Read the model definition and answer for the solid it produces. Units are mm, in the model's axes. A direction names the side the tool comes from. Round coordinates to 2 decimals unless told otherwise and drop trailing zeros. Write each loop counter-clockwise with the first axis right and the second up, starting at its lowest first coordinate (ties: lowest second). Pieces come first, ordered by that corner, then holes.
from build123d import *

# Parameters (mm, degrees)
CROQUIS1_W              = 290
CROQUIS1_H              = 898
CROQUIS1_R              = 6
CROQUIS1_R_2            = 7
CROQUIS1_W_2            = 137.6
CROQUIS1_H_2            = 745.6
SALIENTE_EXTRUIR1_DEPTH = 50.8
REDONDEO1_R             = 5
REDONDEO2_R             = 5


with BuildPart() as part:
    # Croquis1 → Saliente-Extruir1 (new body)
    with BuildSketch(Plane(origin=(0, 0, 0), x_dir=(1, 0, 0), z_dir=(0, 1, 0))):
        with Locations((-145, 449)):
            Rectangle(CROQUIS1_W, CROQUIS1_H)
        with Locations(Location((-273.75, 375.5, 0), (0, 0, 270))):
            Circle(CROQUIS1_R, mode=Mode.SUBTRACT)
        with Locations(Location((-273.75, 522.5, 0), (0, 0, 270))):
            Circle(CROQUIS1_R, mode=Mode.SUBTRACT)
        with Locations(Location((-30.75, 377, 0), (0, 0, 270))):
            Circle(CROQUIS1_R_2, mode=Mode.SUBTRACT)
        with Locations(Location((-30.75, 521, 0), (0, 0, 270))):
            Circle(CROQUIS1_R_2, mode=Mode.SUBTRACT)
        with Locations(Location((-30.75, 167, 0), (0, 0, 270))):
            Circle(CROQUIS1_R_2, mode=Mode.SUBTRACT)
        with Locations(Location((-273.75, 732.5, 0), (0, 0, 90))):
            Circle(CROQUIS1_R, mode=Mode.SUBTRACT)
        with Locations(Location((-273.75, 312.5, 0), (0, 0, 270))):
            Circle(CROQUIS1_R, mode=Mode.SUBTRACT)
        with Locations(Location((-30.75, 311, 0), (0, 0, 270))):
            Circle(CROQUIS1_R_2, mode=Mode.SUBTRACT)
        with Locations(Location((-273.75, 165.5, 0), (0, 0, 270))):
            Circle(CROQUIS1_R, mode=Mode.SUBTRACT)
        with Locations(Location((-30.75, 587, 0), (0, 0, 90))):
            Circle(CROQUIS1_R_2, mode=Mode.SUBTRACT)
        with Locations(Location((-273.75, 585.5, 0), (0, 0, 90))):
            Circle(CROQUIS1_R, mode=Mode.SUBTRACT)
        with Locations(Location((-30.75, 731, 0), (0, 0, 90))):
            Circle(CROQUIS1_R_2, mode=Mode.SUBTRACT)
        with Locations((-145, 449)):
            Rectangle(CROQUIS1_W_2, CROQUIS1_H_2, mode=Mode.SUBTRACT)
    extrude(amount=SALIENTE_EXTRUIR1_DEPTH)

    # Redondeo1
    redondeo1_edges = [part.edges().sort_by_distance(p)[0] for p in [
        (-290, 50.8, -449),
        (-145, 50.8, 0),
        (-76.2, 50.8, -449),
        (-145, 50.8, -821.8),
        (-213.8, 50.8, -449),
        (-145, 50.8, -76.2),
        (0, 50.8, -449),
        (-145, 50.8, -898),
    ]]
    fillet(redondeo1_edges, radius=REDONDEO1_R)

    # Redondeo2
    redondeo2_edges = [part.edges().sort_by_distance(p)[0] for p in [
        (-76.2, 0, -449),
        (-145, 0, -821.8),
        (-213.8, 0, -449),
        (-145, 0, -76.2),
        (-145, 0, 0),
        (-290, 0, -449),
        (-145, 0, -898),
        (0, 0, -449),
    ]]
    fillet(redondeo2_edges, radius=REDONDEO2_R)


solid = part.part
Q1. Section A-A (z = -266) is taken. Determine the outline of the cut face in (x, y), then the cut area to 3 significant figures.
Verdict:
outline: (-290, 5) arc R5 ccw to (-285, 0) - (-218.8, 0) arc R5 ccw to (-213.8, 5) - (-213.8, 45.8) arc R5 ccw to (-218.8, 50.8) - (-285, 50.8) arc R5 ccw to (-290, 45.8) - close; (-76.2, 5) arc R5 ccw to (-71.2, 0) - (-5, 0) arc R5 ccw to (0, 5) - (0, 45.8) arc R5 ccw to (-5, 50.8) - (-71.2, 50.8) arc R5 ccw to (-76.2, 45.8) - close
area: 7,700 mm2
Q2. Determine the mould class of faces 3 (the flat face through (-240, 0, -455)), 4 (the flat face through (-213.8, 25, -444)), 5 (the flat face through (-290, 25, -443)) for opening direction X: pulls with the +X half, pulls with the -X half, needs draft (parallel to the pull), parting line crosses it, or undercut.
Verdict:
face 3: needs draft
face 4: undercut
face 5: pulls with the -X half
Q3. Straight lines are drawn through the part: probe 1 along X at (y, z) = (28, -312.5); probe 2 along X at (y, z) = (14, -522); probe 3 along X at (y, z) = (26.5, -85). For each, find the intervals that lie inside material, in ascending order.
Verdict:
probe 1: x = -290 to -279.75, -267.75 to -213.8, -76.2 to -37.59, -23.91 to 0
probe 2: x = -290 to -279.73, -267.77 to -213.8, -76.2 to -37.68, -23.82 to 0
probe 3: x = -290 to -213.8, -76.2 to 0
Q4. Section B-B (y = 25.5) is taken. State how many separate pieces and enclosed holes the cut face has, then the cut area to 3 significant figures.
Verdict:
separate pieces: 1
enclosed holes: 13
area: 156,000 mm2
Q5. Which of the six approach directions +Z, -Z, +X, -X, +Y, -Y give full straight-line access (tool end or side, diameter ignored) to faces 1 (the flat face through (-146, 25, -821.8)), 2 (the flat face through (-147, 25, -898))?
Verdict:
face 1: +Y, -Y
face 2: -Z, +X, -X, +Y, -Y
Q6. A flat-ended cylindrical pin translates along its axis: pin 1 Ø12.5 at (x, z) = (-30.75, -377) entering from +Y. Find the tip coordinate at first contact, or state that the pin passes through.
Verdict:
pin 1: passes through
